Input: part model. Units: mm. Frame: model coordinates. A direction names the side the tool comes from. Coordinates: 2 decimals unless noted, no trailing zeros. Order: outer loops, then holes, each group sorted by start corner. A loop starts at its lowest first (then second) coordinate and runs counter-clockwise, first axis right, second up. Notation, with made-up numbers: (25.5, -34) - (42.5, -34) arc R23 ccw to (42.5, -13) - close; hole circle Ø6 at (25.5, 21.25). An arc over 180 degrees is marked (long way). One line per question, with ' | ' between items.
from build123d import *

# Parameters (mm, degrees)
SKETCH1_W           = 32.5
SKETCH1_H           = 26.3
BOSS_EXTRUDE1_DEPTH = 3.1
SKETCH2_W           = 3.1
SKETCH2_H           = 26.3
BOSS_EXTRUDE2_DEPTH = 17.9
BOSS_EXTRUDE3_DEPTH = 3.1
FILLET1_R           = 2
SKETCH4_R           = 3
SKETCH4_R_2         = 1.5
CUT_EXTRUDE1_DEPTH  = 3.1
CHAMFER1_SIZE       = 1.5
SKETCH5_R           = 4.95
SKETCH5_R_2         = 1.5
CUT_EXTRUDE2_DEPTH  = 25


with BuildPart() as part:
    # Sketch1 → Boss-Extrude1 (new body)
    with BuildSketch(Plane(origin=(0, 0, 0), x_dir=(1, 0, 0), z_dir=(0, 1, 0))):
        with Locations((16.25, 13.15)):
            Rectangle(SKETCH1_W, SKETCH1_H)
    extrude(amount=BOSS_EXTRUDE1_DEPTH)

    # Sketch2 → Boss-Extrude2 (add)
    with BuildSketch(Plane(origin=(0, 3.1, 0), x_dir=(1, 0, 0), z_dir=(0, 1, 0))):
        with Locations((1.55, 13.15)):
            Rectangle(SKETCH2_W, SKETCH2_H)
    extrude(amount=BOSS_EXTRUDE2_DEPTH)

    # Sketch3 → Boss-Extrude3 (add)
    with BuildSketch(Plane(origin=(3.1, 0, 0), x_dir=(0, 0, -1), z_dir=(1, 0, 0))):
        with BuildLine():
            Line((0, 21), (26.3, 21))
            ThreePointArc((26.3, 21), (13.15, 34.15), (0, 21))
        make_face()
    extrude(amount=-BOSS_EXTRUDE3_DEPTH)

    # Fillet1
    fillet1_edges = [part.edges().sort_by_distance(p)[0] for p in [
        (3.1, 3.1, -13.15),
        (0, 0, -13.15),
        (32.5, 1.55, -26.3),
        (32.5, 1.55, 0),
    ]]
    fillet(fillet1_edges, radius=FILLET1_R)

    # Sketch4 → Cut-Extrude1 (cut)
    with BuildSketch(Plane(origin=(3.1, 0, 0), x_dir=(0, 0, -1), z_dir=(1, 0, 0))):
        with Locations((13.15, 21)):
            Circle(SKETCH4_R)
        with Locations((21.65, 21)):
            Circle(SKETCH4_R_2)
        with Locations((4.65, 21)):
            Circle(SKETCH4_R_2)
    extrude(amount=-CUT_EXTRUDE1_DEPTH, mode=Mode.SUBTRACT)

    # Chamfer1
    chamfer1_edges = [part.edges().sort_by_distance(p)[0] for p in [
        (0, 21, -3.15),
        (3.1, 21, -3.15),
        (0, 21, -20.15),
        (3.1, 21, -20.15),
    ]]
    chamfer(chamfer1_edges, length=CHAMFER1_SIZE)

    # Sketch5 → Cut-Extrude2 (cut)
    with BuildSketch(Plane(origin=(0, 3.1, 0), x_dir=(1, 0, 0), z_dir=(0, 1, 0))):
        with Locations(Location((18.8, 13.15, 0), (0, 0, 270))):
            Circle(SKETCH5_R)
        with Locations(Location((25.8, 21.15, 0), (0, 0, 270))):
            Circle(SKETCH5_R_2)
        with Locations(Location((25.8, 5.15, 0), (0, 0, 270))):
            Circle(SKETCH5_R_2)
        with Locations(Location((11.8, 21.15, 0), (0, 0, 270))):
            Circle(SKETCH5_R_2)
        with Locations(Location((11.8, 5.15, 0), (0, 0, 270))):
            Circle(SKETCH5_R_2)
    extrude(amount=-CUT_EXTRUDE2_DEPTH, mode=Mode.SUBTRACT)


solid = part.part
Item 1: Section A-A on x = 11.8. Return the cut outline in (y, z), and give its area (3 significant figures).
Data:
outline: (0, -26.3) - (3.1, -26.3) - (3.1, -22.65) - (0, -22.65) - close; (0, -19.65) - (3.1, -19.65) - (3.1, -6.65) - (0, -6.65) - close; (0, -3.65) - (3.1, -3.65) - (3.1, 0) - (0, 0) - close | area: 62.9 mm^2
Item 2: Section B-B on z = -13.15. Return the cut outline in (x, y).
Data:
outline: (0, 2) arc R2 ccw to (2, 0) - (13.85, 0) - (13.85, 3.1) - (5.1, 3.1) arc R2 cw to (3.1, 5.1) - (3.1, 18) - (0, 18) - close; (0, 24) - (3.1, 24) - (3.1, 34.15) - (0, 34.15) - close; (23.75, 0) - (32.5, 0) - (32.5, 3.1) - (23.75, 3.1) - close
Item 3: Contact query for flat-ended pins moving along their axis: P1, Ø4, axis at x = 25.8, z = -5.15, coming from the -Y side; P2, Ø1, axis at x = 16, z = -22, coming from the +Y side; P3, Ø10, axis at y = 30.5, z = -12, coming from the +X side. Output: stop coordinate, or through.
Data:
P1: y = 0 | P2: y = 3.1 | P3: x = 3.1
Item 4: Section C-C on x = 18.8. Return the cut outline in (y, z), and give its area (3 significant figures).
Data:
outline: (0, -26.3) - (3.1, -26.3) - (3.1, -18.1) - (0, -18.1) - close; (0, -8.2) - (3.1, -8.2) - (3.1, 0) - (0, 0) - close | area: 50.8 mm^2
Item 5: Ray query, line 1 (X direction, y = 1.9, z = -5.15); line 2 (Z direction, x = 25, y = 1); line 3 (Y direction, x = 30.5, z = -22.75). Return the intervals inside material, ascending.
Data:
line 1: 0 to 10.3, 13.3 to 24.3, 27.3 to 32.5 | line 2: -26.3 to -22.42, -19.88 to -6.42, -3.88 to 0 | line 3: 0 to 3.1
Item 6: Section D-D on z = -4.65. Return the cut outline in (x, y), and give its area (3 significant figures).
Data:
outline: (0, 2) arc R2 ccw to (2, 0) - (10.39, 0) - (10.39, 3.1) - (5.1, 3.1) arc R2 cw to (3.1, 5.1) - (3.1, 18) - (1.6, 19.5) - (1.5, 19.5) - (0, 18) - close; (0, 24) - (1.5, 22.5) - (1.6, 22.5) - (3.1, 24) - (3.1, 31.03) - (0, 31.03) - close; (13.21, 0) - (24.39, 0) - (24.39, 3.1) - (13.21, 3.1) - close; (27.21, 0) - (32.5, 0) - (32.5, 3.1) - (27.21, 3.1) - close | area: 156 mm^2
Item 7: Access query for faces 1 (the face through (10.47, 1.57, -4.46)), 2 (the face through (19, 3.1, -19)). Directions: +Z, -Z, +X, -X, +Y, -Y. A direction counts if a zero-diameter tool reaches every point of the face in a straight line with its end or side. Return the directions, or none.
Data:
face 1: +Y, -Y | face 2: +Z, -Z, +X, +Y
